Autodesk Inventor part; units mm, degrees
ref_plane "YZ Plane" through (0, 0, 0) normal (1, 0, 0) x (0, 1, 0)
ref_plane "XZ Plane" through (0, 0, 0) normal (0, 1, 0) x (-1, 0, 0)
ref_plane "XY Plane" through (0, 0, 0) normal (0, 0, 1) x (1, 0, 0)
sketch "Sketch1" plane through (0, 0, 0) normal (0, 0, 1) x (1, 0, 0)
  line L0 (0, 0) -> (150, 0)
  line L1 (150, 3) -> (0, 3)
  arc A0 (0, 3) -> (0, 0) centre (0, 1.5) ccw
  arc A1 (150, 0) -> (150, 3) centre (150, 1.5) ccw
  circle A2 centre (0, 1.5) radius 1
  circle A3 centre (150, 1.5) radius 1
  line L2 (0, 3) -> (0, 0)
  line L3 (150, 3) -> (150, 0)
  dimension "d2" = 2
  dimension "d3" = 2
  dimension "d9" = 150
extrude "Extrusion1" add sketch "Sketch1" along normal blind 3 contours L2 A2 L1 L3 A3 L0 | A0 L2 A2 | L3 A3 A1
properties part number "L1"
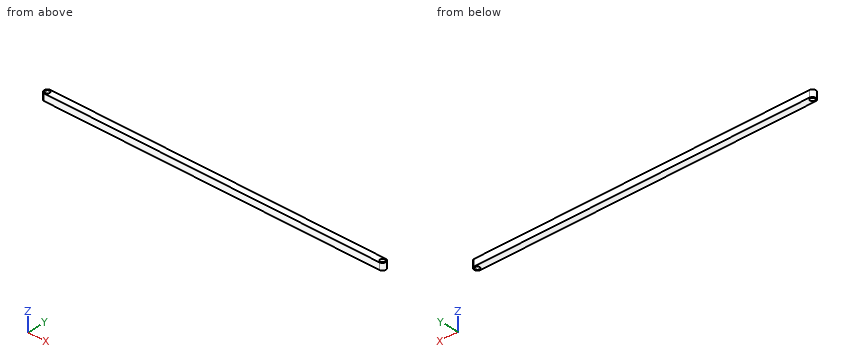
Verification items for the finished model (mm, model axes). Give positions to 0.01 mm unless a question says otherwise; leave off trailing zeros. Write each loop counter-clockwise with the first axis right and the second up, starting at its lowest first coordinate (ties: lowest second). Pieces come first, ordered by that corner, then holes. Notation, with made-up numbers: M 49,1.25 L 76,1.25 A25 cw 76,33.25 Z; hole C 34,56.5 d11. An arc over 180 degrees is marked long. Use CSV: the item, a comma, the result in double quotes.
1) Cross-section at B-B (z = 1.35). Enter the section's corners in (x, y), plus the area to 3 significant figures.
Final values:
outline,"M 0,0 L 150,0 A1.5 ccw 150,3 L 0,3 A1.5 ccw Z; hole C 0,1.5 d2; hole C 150,1.5 d2"
area,"451 mm²"
2) Cross-section at A-A (y = 1.5). Enter the section's corners in (x, z), plus the area to 3 significant figures.
Final values:
outline,"M -1.5,0 L -1,0 L -1,3 L -1.5,3 Z; M 1,0 L 149,0 L 149,3 L 1,3 Z; M 151,0 L 151.5,0 L 151.5,3 L 151,3 Z"
area,"447 mm²"
3) Material ranges on line 1 along X through (y, z) = (1.5, 0.8); line 2 along Y through (x, z) = (0, 1.45); line 3 along X through (y, z) = (1.1, 0.45), recorded low to high.
Final values:
line 1,"-1.5 to -1, 1 to 149, 151 to 151.5"
line 2,"0 to 0.5, 2.5 to 3"
line 3,"-1.45 to -0.92, 0.92 to 149.08, 150.92 to 151.45"
4) Go/stop test with a flat-tipped pin: pin 1 Ø1.2 at (x, y) = (150, 1.5) entering from +Z. Record where the tip stops, or that it passes through.
Final values:
pin 1,"through"
